```python
from build123d import *

# Parameters (mm, degrees)
F1_DEPTH = 7
F2_SIZE  = 1
F3_SIZE  = 1


with BuildPart() as f1:
    # F0 (on Top) → F1 (new body)
    with BuildSketch(Plane.XY):
        with BuildLine():
            ThreePointArc((9.5695807118, 5.525), (10.6734803805, 2.8599504484), (11.05, 0))
            ThreePointArc((11.05, 0), (10.4737971003, -3.5216578911), (8.8052806693, -6.6760416667))
            Line((8.8052806693, -6.6760416667), (11.9840638306, -9.0861509672))
            ThreePointArc((11.9840638306, -9.0861509672), (14.2549292536, -4.7930071218), (15.0391464284, 0))
            ThreePointArc((15.0391464284, 0), (14.5266999405, 3.8924175178), (13.0242828582, 7.5195732142))
            Line((13.0242828582, 7.5195732142), (9.5695807118, 5.525))
        make_face()
        with BuildLine():
            ThreePointArc((0, 11.05), (5.525, 9.5695807118), (9.5695807118, 5.525))
            Line((9.5695807118, 5.525), (13.0242828582, 7.5195732142))
            ThreePointArc((13.0242828582, 7.5195732142), (7.5195732142, 13.0242828582), (0, 15.0391464284))
            Line((0, 15.0391464284), (0, 11.05))
        make_face()
        with BuildLine():
            Line((11.9840638306, -9.0861509672), (8.8052806693, -6.6760416667))
            ThreePointArc((8.8052806693, -6.6760416667), (4.9159047785, -9.8962811302), (0, -11.05))
            Line((0, -11.05), (0, -15.0391464284))
            ThreePointArc((0, -15.0391464284), (6.6905893025, -13.4689249786), (11.9840638306, -9.0861509672))
        make_face()
        with BuildLine():
            ThreePointArc((-9.5695807118, 5.525), (-5.525, 9.5695807118), (0, 11.05))
            Line((0, 11.05), (0, 15.0391464284))
            ThreePointArc((0, 15.0391464284), (-7.5195732142, 13.0242828582), (-13.0242828582, 7.5195732142))
            Line((-13.0242828582, 7.5195732142), (-9.5695807118, 5.525))
        make_face()
        with BuildLine():
            Line((25.1147367097, 14.5), (13.0242828582, 7.5195732142))
            ThreePointArc((13.0242828582, 7.5195732142), (14.5266999405, 3.8924175178), (15.0391464284, 0))
            ThreePointArc((15.0391464284, 0), (14.2549292536, -4.7930071218), (11.9840638306, -9.0861509672))
            Line((11.9840638306, -9.0861509672), (19.2752742891, -14.6142456014))
            Line((19.2752742891, -14.6142456014), (41.5692193817, 24))
            Line((41.5692193817, 24), (16.2788205961, 24))
            ThreePointArc((16.2788205961, 24), (21.2348568775, 19.7504646374), (25.1147367097, 14.5))
        make_face()
        with BuildLine():
            Line((0, -15.0391464284), (0, -11.05))
            ThreePointArc((0, -11.05), (-4.9159047785, -9.8962811302), (-8.8052806693, -6.6760416667))
            Line((-8.8052806693, -6.6760416667), (-11.9840638306, -9.0861509672))
            ThreePointArc((-11.9840638306, -9.0861509672), (-6.6905893025, -13.4689249786), (0, -15.0391464284))
        make_face()
        with BuildLine():
            ThreePointArc((-8.8052806693, -6.6760416667), (-11.028383251, -0.6908421443), (-9.5695807118, 5.525))
            Line((-9.5695807118, 5.525), (-13.0242828582, 7.5195732142))
            ThreePointArc((-13.0242828582, 7.5195732142), (-15.0097258444, -0.9402421871), (-11.9840638306, -9.0861509672))
            Line((-11.9840638306, -9.0861509672), (-8.8052806693, -6.6760416667))
        make_face()
        with BuildLine():
            ThreePointArc((-13.0242828582, 7.5195732142), (-7.5195732142, 13.0242828582), (0, 15.0391464284))
            Line((0, 15.0391464284), (0, 24))
            Line((0, 24), (-41.5692193817, 24))
            Line((-41.5692193817, 24), (-28.9240199889, 2.0978721799))
            ThreePointArc((-28.9240199889, 2.0978721799), (-27.7218325513, 8.514693183), (-25.1147367097, 14.5))
            Line((-25.1147367097, 14.5), (-13.0242828582, 7.5195732142))
        make_face()
        with BuildLine():
            add(Edge.make_bspline(
                [(-16.9558289563, 21.3208617303), (-16.4874368687, 20.9331522104), (-16.4874368687, 20.165314083)],
                knots=[0, 0, 0, 1, 1, 1], degree=2))
            add(Edge.make_bspline(
                [(-16.4874368687, 20.165314083), (-16.4874368687, 19.3660693185), (-16.9866940996, 18.9431627053)],
                knots=[0, 0, 0, 1, 1, 1], degree=2))
            add(Edge.make_bspline(
                [(-16.9866940996, 18.9431627053), (-17.4859513306, 18.5202560921), (-18.4064906935, 18.5202560921)],
                knots=[0, 0, 0, 1, 1, 1], degree=2))
            Line((-18.4064906935, 18.5202560921), (-18.8559305, 18.5202560921))
            Line((-18.8559305, 18.5202560921), (-18.8559305, 16.7604014277))
            Line((-18.8559305, 16.7604014277), (-19.9053453737, 16.7604014277))
            Line((-19.9053453737, 16.7604014277), (-19.9053453737, 21.7085712502))
            Line((-19.9053453737, 21.7085712502), (-18.325266632, 21.7085712502))
            add(Edge.make_bspline(
                [(-18.325266632, 21.7085712502), (-17.4242210439, 21.7085712502), (-16.9558289563, 21.3208617303)],
                knots=[0, 0, 0, 1, 1, 1], degree=2))
        make_face(mode=Mode.SUBTRACT)
        Polygon((-11.3930637356, 16.7604014277), (-12.5237026708, 16.7604014277), (-12.8821715286, 17.9386918123), (-14.6864286799, 17.9386918123), (-15.0448975376, 16.7604014277), (-16.1755364728, 16.7604014277), (-14.4286776582, 21.7291480124), (-13.1464204751, 21.7291480124), align=None, mode=Mode.SUBTRACT)
        with BuildLine():
            Line((-7.788881383, 21.7085712502), (-6.7427154718, 21.7085712502))
            Line((-6.7427154718, 21.7085712502), (-6.7427154718, 18.5072602423))
            add(Edge.make_bspline(
                [(-6.7427154718, 18.5072602423), (-6.7427154718, 17.958185587), (-6.9880121373, 17.5455673549)],
                knots=[0, 0, 0, 1, 1, 1], degree=2))
            add(Edge.make_bspline(
                [(-6.9880121373, 17.5455673549), (-7.2333088028, 17.1329491228), (-7.6973689405, 16.9125611695)],
                knots=[0, 0, 0, 1, 1, 1], degree=2))
            add(Edge.make_bspline(
                [(-7.6973689405, 16.9125611695), (-8.1614290781, 16.6921732161), (-8.7938937698, 16.6921732161)],
                knots=[0, 0, 0, 1, 1, 1], degree=2))
            add(Edge.make_bspline(
                [(-8.7938937698, 16.6921732161), (-9.7480057448, 16.6921732161), (-10.2759621441, 17.1816835597)],
                knots=[0, 0, 0, 1, 1, 1], degree=2))
            add(Edge.make_bspline(
                [(-10.2759621441, 17.1816835597), (-10.8039185434, 17.6711939033), (-10.8039185434, 18.5202560921)],
                knots=[0, 0, 0, 1, 1, 1], degree=2))
            Line((-10.8039185434, 18.5202560921), (-10.8039185434, 21.7085712502))
            Line((-10.8039185434, 21.7085712502), (-9.7588356196, 21.7085712502))
            Line((-9.7588356196, 21.7085712502), (-9.7588356196, 18.6794552525))
            add(Edge.make_bspline(
                [(-9.7588356196, 18.6794552525), (-9.7588356196, 18.10763786), (-9.5287007789, 17.8401399511)],
                knots=[0, 0, 0, 1, 1, 1], degree=2))
            add(Edge.make_bspline(
                [(-9.5287007789, 17.8401399511), (-9.2985659382, 17.5726420421), (-8.7668190827, 17.5726420421)],
                knots=[0, 0, 0, 1, 1, 1], degree=2))
            add(Edge.make_bspline(
                [(-8.7668190827, 17.5726420421), (-8.2524000269, 17.5726420421), (-8.020640705, 17.8417644323)],
                knots=[0, 0, 0, 1, 1, 1], degree=2))
            add(Edge.make_bspline(
                [(-8.020640705, 17.8417644323), (-7.788881383, 18.1108868225), (-7.788881383, 18.6859531774)],
                knots=[0, 0, 0, 1, 1, 1], degree=2))
            Line((-7.788881383, 18.6859531774), (-7.788881383, 21.7085712502))
        make_face(mode=Mode.SUBTRACT)
        Polygon((-2.4746617904, 16.7604014277), (-5.5308524752, 16.7604014277), (-5.5308524752, 21.7085712502), (-4.4814376015, 21.7085712502), (-4.4814376015, 17.6267914164), (-2.4746617904, 17.6267914164), align=None, mode=Mode.SUBTRACT)
        with BuildLine():
            Line((0, -29), (0, -15.0391464284))
            ThreePointArc((0, -15.0391464284), (-6.6905893025, -13.4689249786), (-11.9840638306, -9.0861509672))
            Line((-11.9840638306, -9.0861509672), (-19.2752742891, -14.6142456014))
            Line((-19.2752742891, -14.6142456014), (0, -48))
            Line((0, -48), (12.6451993928, -26.0978721799))
            ThreePointArc((12.6451993928, -26.0978721799), (6.4869756738, -28.2651578203), (0, -29))
        make_face()
    extrude(amount=F1_DEPTH)

    # F2
    f2_edges = [f1.edges().sort_by_distance(p)[0] for p in [
        (-20.78461, 24, 7),
        (-35.24662, 13.048936, 7),
        (-19.06951, 11.009787, 7),
        (-15.009726, -0.940242, 7),
        (-27.721833, 8.514693, 7),
        (-15.629669, -11.850198, 7),
        (-9.637637, -31.307123, 7),
        (6.3226, -37.048936, 7),
        (6.690589, -13.468925, 7),
        (0, -22.019573, 7),
        (6.486976, -28.265158, 7),
        (15.629669, -11.850198, 7),
        (30.422247, 4.692877, 7),
        (28.92402, 24, 7),
        (21.234857, 19.750465, 7),
        (19.06951, 11.009787, 7),
        (7.519573, 13.024283, 7),
        (0, 19.519573, 7),
    ]]
    chamfer(f2_edges, length=F2_SIZE)

    # F3
    f3_edges = [f1.edges().sort_by_distance(p)[0] for p in [
        (-9.637637, -31.307123, 0),
        (6.3226, -37.048936, 0),
        (0, -22.019573, 0),
        (6.486976, -28.265158, 0),
        (6.690589, -13.468925, 0),
        (15.629669, -11.850198, 0),
        (30.422247, 4.692877, 0),
        (28.92402, 24, 0),
        (21.234857, 19.750465, 0),
        (19.06951, 11.009787, 0),
        (7.519573, 13.024283, 0),
        (0, 19.519573, 0),
        (-20.78461, 24, 0),
        (-35.24662, 13.048936, 0),
        (-27.721833, 8.514693, 0),
        (-19.06951, 11.009787, 0),
        (-15.009726, -0.940242, 0),
        (-15.629669, -11.850198, 0),
    ]]
    chamfer(f3_edges, length=F3_SIZE)


solid = f1.part
```
Can you work these out from the model? Positions are in its coordinate system, mm. A direction names the side the tool comes from. Round coordinates to 2 decimals unless told otherwise and drop trailing zeros. Loops run counter-clockwise (first coordinate to the right, second up) from the corner with the lowest first, then second, coordinate; pieces in that order, holes last.
Item 1: Will these pins go through, and if not, where does the flat tip stop? pin 1 Ø1.5 at (y, z) = (20.5, 3.5) entering from -X; pin 2 Ø3 at (y, z) = (-30, 1.5) entering from -X; pin 3 Ø1.7 at (x, z) = (-19, 2) entering from -Y.
Item 2: Suppose I cut it at B-B, the plane y = -31.5. Write out the boundary of the cut face in (x, z), then the cut area to 3 significant figures.
Item 3: Which directions (+Z, -Z, +X, -X, +Y, -Y) give clear straight access to the entire face, cutting with the end or side of a thin tool? Please do faces 1 (the flat face through (-19.905, 19, 3)), 2 (the conical face through (6.228, -12.776, 0.174)), 3 (the cylindrical face through (7.61, 12.97, 3.47)), 4 (the conical face through (-14.18, -0.76, 6.84)).
Item 4: Suppose I cut it at A-A, the plane z = 5. State how many separate pieces and enclosed holes the cut face has, then the cut area to 3 significant figures.
Item 5: Please list where these lines run through material, in increasing order: L1, parallel to Y at x = 6, z = 6.25; L2, parallel to Y at x = 23, z = 5.25; L3, parallel to X at y = 16.5, z = 2.25.
Item 6: If we mould it in two halves opening along Y, with no side actions, what happens to faces 5 (the flat face through (-19.154, 11.059, 3.465)), 6 (the flat face through (-20, 24, 3)), 7 (the conical face through (-14.18, -0.76, 0.16)), 8 (the flat face through (-9.773, -31.073, 3.465))? For each: +Y half, -Y half, draft (parallel to the pull), parting line (faces both ways), or undercut.
Reported:
1. pin 1: stops at x = -39.98
1. pin 2: stops at x = -11.26
1. pin 3: stops at y = -16.56
2. outline: (-9.53, 1) - (-8.37, 0) - (8.37, 0) - (9.53, 1) - (9.53, 6) - (8.37, 7) - (-8.37, 7) - (-9.53, 6) - close
2. area: 131 mm2
3. face 1: +Z, -Z
3. face 2: -Z
3. face 3: +Z, -Z, +Y
3. face 4: +Z
4. separate pieces: 1
4. enclosed holes: 5
4. area: 1,770 mm2
5. L1: y = -37.11 to -28.63, -13.52 to -9.28, 9.28 to 13.52
5. L2: y = -8.16 to 13.28, 17.66 to 24
5. L3: x = -37.24 to 0, 23.85 to 37.24
6. face 5: undercut
6. face 6: +Y half
6. face 7: undercut
6. face 8: -Y half
